```python
from build123d import *

# Parameters (mm, degrees)
BOSS_EXTRUDE1_DEPTH    = 9.6
SKETCH2_OUTSIDE_W      = 73.45
SKETCH2_OUTSIDE_H      = 69.428
SKETCH2_OUTSIDE_R      = 13
CUT_EXTRUDE1_DEPTH     = 9.6
CUT_EXTRUDE1_DRAFT     = -60
SKETCH3_OUTSIDE_W      = 73.45
SKETCH3_OUTSIDE_H      = 69.428
SKETCH3_OUTSIDE_R      = 13
CUT_EXTRUDE2_DEPTH     = 9.6
CUT_EXTRUDE2_DRAFT     = -60
M12_TAPPED_HOLE1_D     = 10.2
M12_TAPPED_HOLE1_DEPTH = 32.75
CHAMFER1_SIZE          = 0.5


with BuildPart() as part:
    # Sketch1 → Boss-Extrude1 (new body)
    with BuildSketch(Plane(origin=(0, 0, 0), x_dir=(1, 0, 0), z_dir=(0, 1, 0))):
        Polygon((15.011106999, 0), (7.505553499, 13), (-7.505553499, 13), (-15.011106999, 0), (-7.505553499, -13), (7.505553499, -13), align=None)
    extrude(amount=BOSS_EXTRUDE1_DEPTH)


with BuildPart() as cut_extrude1_tool:
    # Sketch2 outside → Cut-Extrude1 (with draft: the straight prism first)
    with BuildSketch(Plane(origin=(0, 9.6, 0), x_dir=(1, 0, 0), z_dir=(0, 1, 0))):
        Rectangle(SKETCH2_OUTSIDE_W, SKETCH2_OUTSIDE_H)
        Circle(SKETCH2_OUTSIDE_R, mode=Mode.SUBTRACT)
    extrude(amount=-CUT_EXTRUDE1_DEPTH)
    # Cut-Extrude1: the draft: its side faces are tilted about the plane it starts from
    cut_extrude1_sides = [cut_extrude1_tool.faces().sort_by_distance(p)[0] for p in [
        (0, 4.8, 34.714),
        (36.725, 4.8, 0),
        (0, 4.8, -34.714),
        (-36.725, 4.8, 0),
        (-13, 4.8, 0),
    ]]
    draft(cut_extrude1_sides, Plane(origin=(0, 9.6, 0), x_dir=(1, 0, 0), z_dir=(0, 1, 0)), CUT_EXTRUDE1_DRAFT)


with BuildPart() as part_1:
    add(part.part)

    # Cut-Extrude1: cut by cut_extrude1_tool
    add(cut_extrude1_tool.part, mode=Mode.SUBTRACT)


with BuildPart() as cut_extrude2_tool:
    # Sketch3 outside → Cut-Extrude2 (with draft: the straight prism first)
    with BuildSketch(Plane.XZ):
        Rectangle(SKETCH3_OUTSIDE_W, SKETCH3_OUTSIDE_H)
        Circle(SKETCH3_OUTSIDE_R, mode=Mode.SUBTRACT)
    extrude(amount=-CUT_EXTRUDE2_DEPTH)
    # Cut-Extrude2: the draft: its side faces are tilted about the plane it starts from
    cut_extrude2_sides = [cut_extrude2_tool.faces().sort_by_distance(p)[0] for p in [
        (0, 4.8, -34.714),
        (36.725, 4.8, 0),
        (0, 4.8, 34.714),
        (-36.725, 4.8, 0),
        (-13, 4.8, 0),
    ]]
    draft(cut_extrude2_sides, Plane.XZ, CUT_EXTRUDE2_DRAFT)


with BuildPart() as part_2:
    add(part_1.part)

    # Cut-Extrude2: cut by cut_extrude2_tool
    add(cut_extrude2_tool.part, mode=Mode.SUBTRACT)

    # M12 Tapped Hole1
    with Locations(Plane(origin=(0, 9.6, 0), x_dir=(1, 0, 0), z_dir=(0, 1, 0))):
        with Locations((0, 0)):
            Hole(M12_TAPPED_HOLE1_D / 2, depth=M12_TAPPED_HOLE1_DEPTH)

    # Chamfer1
    chamfer1_edges = [part_2.edges().sort_by_distance(p)[0] for p in [
        (5.1, 0, 0),
        (5.1, 9.6, 0),
    ]]
    chamfer(chamfer1_edges, length=CHAMFER1_SIZE)


solid = part_2.part
```
The model under review builds one solid part; all positions refer to its coordinate system, in mm. Round coordinates to 2 decimals unless told otherwise and drop trailing zeros. Order: outer loops, then holes, each group sorted by start corner. A loop starts at its lowest first (then second) coordinate and runs counter-clockwise, first axis right, second up.
(1) For P1, Ø1.5, axis at x = 9.5, y = 3.5, coming from the +Z side; P2, Ø3, axis at y = 5.5, z = 6, coming from the -X side, all flat-tipped, find the tip position at first contact; note any pin that passes through.
Working result:
P1: stops at z = 10.84
P2: stops at x = -12.41
(2) Wall thickness on L1, parallel to Z at x = 0, y = 5; L2, parallel to X at y = 1.25, z = 1.25; L3, parallel to X at y = 4.5, z = -5.5: over which ranges is each line inside the solid? List them lowest first.
Working result:
L1: z = -13 to -5.1, 5.1 to 13
L2: x = -14.29 to -4.94, 4.94 to 14.29
L3: x = -11.84 to 11.84
(3) Mouldability with a two-part tool opening along X and no side actions: class faces 1 (the face through (6.77, 9.32, -11.66)), 2 (the face through (-2.4, 4.7, 4.5)), 3 (the face through (0, 5, -13)) as released by +X, released by -X, zero draft, split by the parting line, or undercut.
Working result:
face 1: released by +X
face 2: undercut
face 3: zero draft
(4) Take a section at A-A, the plane y = 2.25. State the section outline as (x, z) points.
Working result:
outline: (-15.01, 0) - (-7.51, -13) - (7.51, -13) - (15.01, 0) - (7.51, 13) - (-7.51, 13) - close; hole circle Ø10.2 at (0, 0)
